Input: part model. Units: mm. Frame: model coordinates. Face numbers are marked on the shaded views. A direction names the side the tool comes from. Round coordinates to 2 decimals unless told otherwise and drop trailing zeros. Loops run counter-clockwise (first coordinate to the right, second up) from the corner with the lowest first, then second, coordinate; pieces in that order, holes last. Notation, with made-up numbers: (1, 31.25) -> (42, 31.25) arc R15 ccw to (42, 47.25) -> close; hole circle Ø4 at (24.5, -19). An arc over 180 degrees is marked (long way). Answer in a Markdown table with one row per item. Add a question column.
Q1. Ray query, L1, parallel to Y at x = 0, z = 1.5; L2, parallel to X at y = 7, z = -1.25; L3, parallel to Z at x = 0, y = 14. Return the intervals inside material, ascending. Write a range as from..to.
Q2. Section D-D, the plane x = 8. Give the number of separate pieces and of enclosed holes in the cut face, and give its area (3 significant figures).
Q3. Reachability of the marked faces 5, 6, 7, 8 and 9 from +Z, -Z, +X, -X, +Y, -Y: full face, straight path, thin tool, end or side. Return the list, or none.
Q4. Pin query (flat end, axial travel): pin 1 (1.5 mm diameter, centred on x = -12.5, z = -2, fed in from -Y); pin 2 (5 mm diameter, centred on y = 0, z = 0, fed in from -X); pin 3 (12 mm diameter, centred on x = 3.5, y = 9.5, fed in from +Z); pin 4 (5 mm diameter, centred on x = 0, z = 0, fed in from +Y). Return the tip coordinate at first contact, or that it passes through.
Q5. Mould query, pull axis Z, two halves, no side actions, for the marked faces 1, 2, 3 and 4. Classes: pulls with the +Z half, pulls with the -Z half, needs draft (parallel to the pull), parting line crosses it, or undercut.
Q6. Section C-C, the plane y = -5.5. Output: boundary loops of the cut face in (x, z), and give its area (3 significant figures).
Q7. Section A-A, the plane y = 0. Output: boundary loops of the cut face in (x, z).
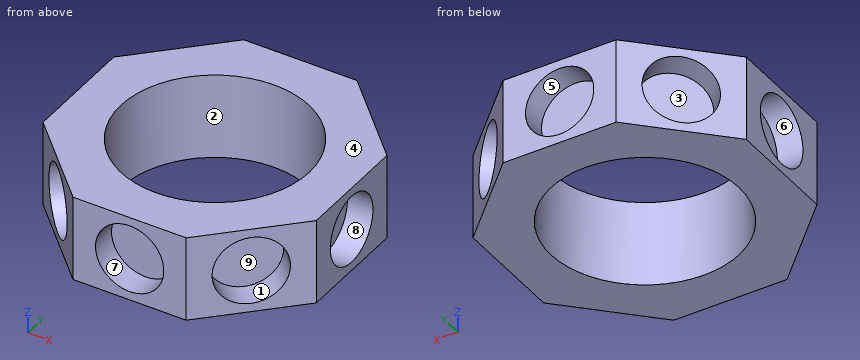
```python
from build123d import *

# Parameters (mm, degrees)
SKETCH1_R           = 11
BOSS_EXTRUDE1_DEPTH = 5
SKETCH2_R           = 4
CUT_EXTRUDE3_DEPTH  = 3
CIRPATTERN1_COUNT   = 8


with BuildPart() as part:
    # Sketch1 → Boss-Extrude1 (new body, symmetric)
    with BuildSketch(Plane.XY):
        Polygon((6.627416998, 16), (-6.627416998, 16), (-16, 6.627416998), (-16, -6.627416998), (-6.627416998, -16), (6.627416998, -16), (16, -6.627416998), (16, 6.627416998), align=None)
        Circle(SKETCH1_R, mode=Mode.SUBTRACT)
    extrude(amount=BOSS_EXTRUDE1_DEPTH, both=True)

    # Sketch2 → Cut-Extrude3 (cut)
    with BuildSketch(Plane(origin=(0, -16, 0), x_dir=(-1, 0, 0), z_dir=(0, -1, 0))):
        Circle(SKETCH2_R)
    cut_extrude3 = extrude(amount=-CUT_EXTRUDE3_DEPTH, mode=Mode.SUBTRACT)

    # CirPattern1: Cut-Extrude3 ×8 about axis
    cirpattern1_axis = Axis((0, 0, 0), (0, 0, 1))
    for i in range(1, CIRPATTERN1_COUNT):
        add(cut_extrude3.rotate(cirpattern1_axis, i * 360 / CIRPATTERN1_COUNT), mode=Mode.SUBTRACT)


solid = part.part
```
Answer block:
| question | item | result |
|---|---|---|
| 1 | L1 | -13..-11, 11..13 |
| 1 | L2 | -15.63..-12.37, -11.38..-8.49, 8.49..11.38, 12.37..15.63 |
| 1 | L3 | -5..-4, 4..5 |
| 2 | separate pieces | 2 |
| 2 | enclosed holes | 2 |
| 2 | area | 107 mm^2 |
| 3 | face 5 | +Y |
| 3 | face 6 | -X |
| 3 | face 7 | -Y |
| 3 | face 8 | +X |
| 3 | face 9 | none |
| 4 | pin 1 | y = -8.65 |
| 4 | pin 2 | x = -13 |
| 4 | pin 3 | z = 5 |
| 4 | pin 4 | y = 13 |
| 5 | face 1 | undercut |
| 5 | face 2 | needs draft |
| 5 | face 3 | undercut |
| 5 | face 4 | pulls with the +Z half |
| 6 | outline | (-16, -5) -> (-9.53, -5) -> (-9.53, 5) -> (-16, 5) -> close; (9.53, -5) -> (16, -5) -> (16, 5) -> (9.53, 5) -> close |
| 6 | area | 129 mm^2 |
| 7 | outline | (-16, -5) -> (-11, -5) -> (-11, 5) -> (-16, 5) -> (-16, 4) -> (-13, 4) -> (-13, -4) -> (-16, -4) -> close; (11, -5) -> (16, -5) -> (16, -4) -> (13, -4) -> (13, 4) -> (16, 4) -> (16, 5) -> (11, 5) -> close |
